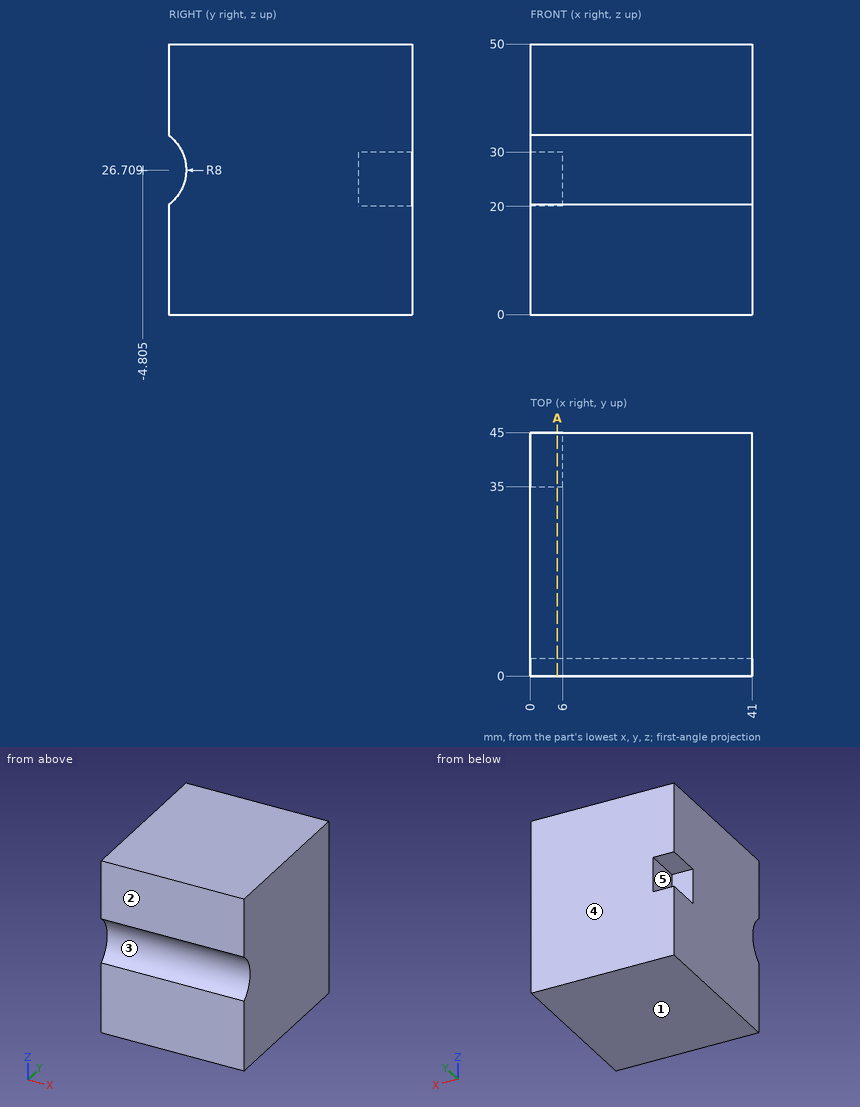
Here's the drawing with two shaded views (mm, measured from the low corner). I have some questions. A direction names the side the tool comes from. Coordinates: 2 decimals unless noted, no trailing zeros. Loops run counter-clockwise (first coordinate to the right, second up) from the corner with the lowest first, then second, coordinate; pieces in that order, holes last.
Item 1: Which directions (+Z, -Z, +X, -X, +Y, -Y) give clear straight access to the entire face, cutting with the end or side of a thin tool? Please do the marked faces 4 and 5.
Answers below:
face 4: +Z, -Z, +X, -X, +Y
face 5: -X, +Y
Item 2: Please list where these lines run through material, in increasing order: L1, parallel to Y at x = 10.5, z = 22 (1 decimal); L2, parallel to Y at x = 27, z = 25.
Answers below:
L1: y = 1.7 to 45
L2: y = 3.01 to 45
Item 3: Suppose I cut it at A-A (x = 5). Please give me the cut outline in (y, z) (1 decimal), then the cut area to 3 significant figures.
Answers below:
outline: (0, 0) - (45, 0) - (45, 20) - (35, 20) - (35, 30) - (45, 30) - (45, 50) - (0, 50) - (0, 33.1) arc R8 cw to (0, 20.3) - close
area: 2,120 mm2
Item 4: I'm going to push flat-ended pins straight in: pin 1 (1.8 mm diameter, centred on x = 2.5, z = 25.5, fed in from +Y); pin 2 (5 mm diameter, centred on y = 41, z = 26.5, fed in from -X). Where does each tip first touch, or does it pass through?
Answers below:
pin 1: stops at y = 35
pin 2: stops at x = 6
Item 5: If we mould it in two halves opening along Z, with no side actions, what happens to the marked faces 1, 2 and 3? For each: released by +Z, released by -Z, zero draft, split by the parting line, or undercut.
Answers below:
face 1: released by -Z
face 2: zero draft
face 3: undercut
